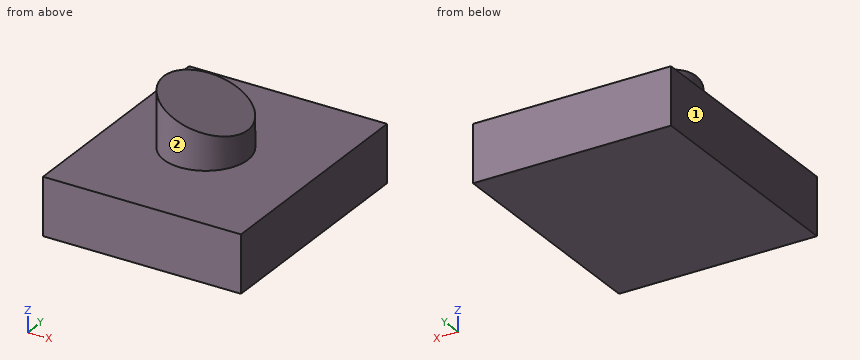
```python
from build123d import *

# Parameters (mm, degrees)
F0_W     = 87.957568
F0_H     = 104.53599
F1_DEPTH = 25.4
F2_R     = 18.659925
F3_DEPTH = 25.4
F5_DEPTH = 104.536989


with BuildPart() as f1:
    # F0 (on Top) → F1 (new body)
    with BuildSketch(Plane.XY):
        Rectangle(F0_W, F0_H)
    extrude(amount=F1_DEPTH)

    # F2 (on face) → F3 (join)
    with BuildSketch(Plane.XY.offset(25.4)):
        with Locations((-4.059047, 0)):
            Circle(F2_R)
    extrude(amount=F3_DEPTH)

    # F4 (on face) → F5 (cut, through all)
    with BuildSketch(Plane.XZ.offset(52.267995)):
        Polygon((14.600879, 50.8), (-22.718972, 50.8), (14.600879, 38.1), align=None)
    extrude(amount=-F5_DEPTH, mode=Mode.SUBTRACT)


solid = f1.part
```
Work out the finished part from the listing and answer in its coordinate system (mm). Face numbers are marked on the shaded views. A direction names the side the tool comes from. Coordinates: 2 decimals unless noted, no trailing zeros. Write each loop counter-clockwise with the first axis right and the second up, starting at its lowest first coordinate (ties: lowest second). Pieces come first, ordered by that corner, then holes.
Q1. Each of these flat-tipped pins is pushed along its axis until it touches: pin 1 Ø5 at (x, z) = (-11, 32) entering from -Y; pin 2 Ø1.5 at (x, z) = (12, 35) entering from +Y; pin 3 Ø10 at (x, y) = (-26, 7) entering from +Z. Where does it stop, or does it pass through?
Q2. A cutting plane is placed at A-A, the plane y = 0. Give the vertices of the cut face in (x, z).
Q3. A cutting plane is placed at D-D, the plane y = 37. Give the vertices of the cut face in (x, z), then the cut area to 3 significant figures.
Q4. Which of the six approach directions +Z, -Z, +X, -X, +Y, -Y give full straight-line access (tool end or side, diameter ignored) to the marked faces 1 and 2?
Q5. A cutting plane is placed at B-B, the plane x = -5.5. Give the vertices of the cut face in (y, z), then the cut area to 3 significant figures.
Q6. A cutting plane is placed at C-C, the plane x = 27. Give the vertices of the cut face in (y, z).
Q7. Find the intervals of material crossed by line 1 (Z direction, x = 18.5, y = 25); line 2 (Y direction, x = -8, z = 26); line 3 (Y direction, x = 6, z = 32), in increasing order.
Findings below:
1. pin 1: stops at y = -18.12
1. pin 2: stops at y = 10.67
1. pin 3: stops at z = 50.68
2. outline: (-43.98, 0) - (43.98, 0) - (43.98, 25.4) - (14.6, 25.4) - (14.6, 38.1) - (-22.72, 50.8) - (-22.72, 25.4) - (-43.98, 25.4) - close
3. outline: (-43.98, 0) - (43.98, 0) - (43.98, 25.4) - (-43.98, 25.4) - close
3. area: 2,230 mm2
4. face 1: +Z, -Z, -X, +Y, -Y
4. face 2: +Z
5. outline: (-52.27, 0) - (52.27, 0) - (52.27, 25.4) - (18.6, 25.4) - (18.6, 44.94) - (-18.6, 44.94) - (-18.6, 25.4) - (-52.27, 25.4) - close
5. area: 3,380 mm2
6. outline: (-52.27, 0) - (52.27, 0) - (52.27, 25.4) - (-52.27, 25.4) - close
7. line 1: z = 0 to 25.4
7. line 2: y = -18.24 to 18.24
7. line 3: y = -15.72 to 15.72
